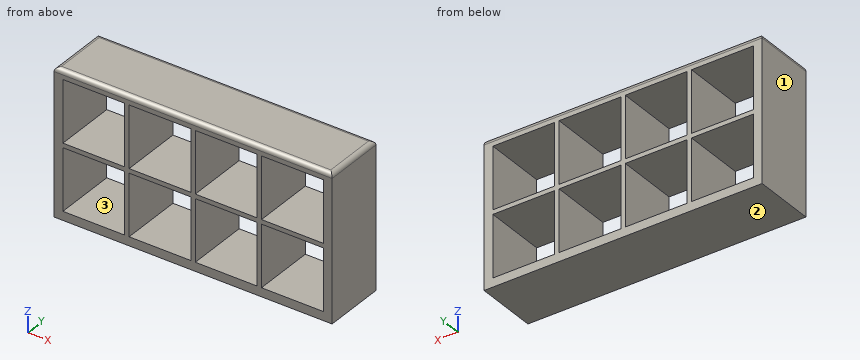
```python
from build123d import *

# Parameters (mm, degrees)
F0_W     = 80.01
F0_H     = 41.91
F0_W_2   = 17.78
F0_H_2   = 17.78
F1_DEPTH = 17.78
F2_R     = 1.27


with BuildPart() as f1:
    # F0 (on Front) → F1 (new body)
    with BuildSketch(Plane.XZ):
        with Locations((-0.565825, 25.926393)):
            Rectangle(F0_W, F0_H)
        with Locations((-29.140825, 16.401393)):
            Rectangle(F0_W_2, F0_H_2, mode=Mode.SUBTRACT)
        with Locations((-10.090825, 16.401393)):
            Rectangle(F0_W_2, F0_H_2, mode=Mode.SUBTRACT)
        with Locations((8.959175, 16.401393)):
            Rectangle(F0_W_2, F0_H_2, mode=Mode.SUBTRACT)
        with Locations((28.009175, 16.401393)):
            Rectangle(F0_W_2, F0_H_2, mode=Mode.SUBTRACT)
        with Locations((-29.140825, 35.451393)):
            Rectangle(F0_W_2, F0_H_2, mode=Mode.SUBTRACT)
        with Locations((-10.090825, 35.451393)):
            Rectangle(F0_W_2, F0_H_2, mode=Mode.SUBTRACT)
        with Locations((8.959175, 35.451393)):
            Rectangle(F0_W_2, F0_H_2, mode=Mode.SUBTRACT)
        with Locations((28.009175, 35.451393)):
            Rectangle(F0_W_2, F0_H_2, mode=Mode.SUBTRACT)
    extrude(amount=F1_DEPTH)

    # F2
    f2_edges = [f1.edges().sort_by_distance(p)[0] for p in [
        (39.439175, -8.89, 46.881393),
        (-40.570825, -8.89, 46.881393),
        (-0.565825, 0, 46.881393),
        (-0.565825, -17.78, 46.881393),
    ]]
    fillet(f2_edges, radius=F2_R)


solid = f1.part
```
Part model, mm, in its own coordinate system. Face numbers are marked on the shaded views. Round coordinates to 2 decimals unless told otherwise and drop trailing zeros. Write each loop counter-clockwise with the first axis right and the second up, starting at its lowest first coordinate (ties: lowest second). Pieces come first, ordered by that corner, then holes. Notation, with made-up numbers: M 17,37 L 37,37 A33 ccw 37,73 Z; hole C -16.75,15 d11. An arc over 180 degrees is marked long. Answer as CSV lines item,"result". Start each with the question number.
1) Band-saw the part on C-C (y = -12). Count the separate pieces of the cut face and the enclosed holes in it, then the cut area to 4 significant figures.
2) Band-saw the part on B-B (z = 21.5). List the corners of the cut face in (x, y), then the cut area to 3 significant figures.
3) Band-saw the part on A-A (x = -2.5). List the corners of the cut face in (y, z).
4) Drill centre lines: L1, parallel to X at y = -13.75, z = 24; L2, parallel to Z at x = 8.5, y = -6.5. Where is each one in solid material? Low to high.
5) Mould opens along X. For the marked faces 1, 2 and 3 say: +X half, -X half, draft (parallel to the pull), parting line (faces both ways), or undercut.
Worked out:
1,separate pieces,"1"
1,enclosed holes,"8"
1,area,"823.5 mm²"
2,outline,"M -40.57,-17.78 L -38.03,-17.78 L -38.03,0 L -40.57,0 Z; M -20.25,-17.78 L -18.98,-17.78 L -18.98,0 L -20.25,0 Z; M -1.2,-17.78 L 0.07,-17.78 L 0.07,0 L -1.2,0 Z; M 17.85,-17.78 L 19.12,-17.78 L 19.12,0 L 17.85,0 Z; M 36.9,-17.78 L 39.44,-17.78 L 39.44,0 L 36.9,0 Z"
2,area,"158 mm²"
3,outline,"M -17.78,4.97 L 0,4.97 L 0,7.51 L -17.78,7.51 Z; M -17.78,25.29 L 0,25.29 L 0,26.56 L -17.78,26.56 Z; M -17.78,44.34 L 0,44.34 L 0,45.61 A1.27 ccw -1.27,46.88 L -16.51,46.88 A1.27 ccw -17.78,45.61 Z"
4,L1,"-40.57 to -38.03, -20.25 to -18.98, -1.2 to 0.07, 17.85 to 19.12, 36.9 to 39.44"
4,L2,"4.97 to 7.51, 25.29 to 26.56, 44.34 to 46.88"
5,face 1,"-X half"
5,face 2,"draft"
5,face 3,"undercut"
